Build history of the part. All positions in model axes, mm. A direction names the side the tool comes from. Give positions to 0.01 mm unless a question says otherwise; leave off trailing zeros. Order: outer loops, then holes, each group sorted by start corner. A loop starts at its lowest first (then second) coordinate and runs counter-clockwise, first axis right, second up. Notation, with made-up numbers: (24, 81.5) - (65, 81.5) arc R24 cw to (65, 119.5) - close; hole circle Ø4 at (79, 44.25). An arc over 180 degrees is marked (long way). Use a Markdown table: item, result. Add a question column.
(1) Slice it at A-A (y = 0). Write the cut outline in (x, z).
(2) Slice it at C-C (z = -12). Write the cut outline in (x, y), then the cut area to 3 significant figures.
(3) Wall check: line 1 (Y direction, x = 0, z = -9.5); line 2 (Z direction, x = -30.5, y = -13); line 3 (Y direction, x = 5.5, z = -12.25). Give the ranges that are in metal, low to high.
(4) Which spindle directions (+Z, -Z, +X, -X, +Y, -Y) get a long thin tool onto all of the face, cutting with end or side? Do faces 5 (the face through (-14, -28, -18.5)), 6 (the face through (22.41, 17.47, 1.93)). Say none if no direction does.
(5) Mould opens along X. For faces 1 (the face through (-25.39, -25.52, -16.04)), 2 (the face through (36, 0, -16)), 3 (the face through (-4.81, 21.15, 5.5)), 4 (the face through (-23.866, -16.582, 1.873)) say: +X half, -X half, draft (parallel to the pull), parting line (faces both ways), or undercut.
(6) Flat gauge pins, fed straight in: pin 1 (4 mm diameter, centred on x = -33.26, y = -13.78, fed in from +Z); pin 2 (1.8 mm diameter, centred on x = -13.78, y = 33.26, fed in from +Z); pin 3 (4 mm diameter, centred on y = 16, z = -1.5, fed in from -X); pin 4 (8 mm diameter, centred on y = -17, z = 2.5, fed in from +X). Where does each tip first touch, or does it go through?
from build123d import *

# Parameters (mm, degrees)
SKETCH_2_R                = 32.5
SKETCH_2_R_2              = 1.5
SKETCH_2_R_3              = 21
EXTRUDE_1_DEPTH           = 5.5
SKETCH_3_R                = 32.5
SKETCH_3_R_2              = 30.5
EXTRUDE_2_DEPTH           = 18.5
SKETCH_4_R                = 1.5
SKETCH_4_R_2              = 30.5
EXTRUDE_3_DEPTH           = 5.5
CHAMFER_1_SIZE            = 1
CHAMFER_3_SIZE            = 0.5
HOLE_WIZARD_0_D           = 3.2
HOLE_WIZARD_0_DEPTH       = 8.1
HOLE_WIZARD_0_CSINK_D     = 6.6
HOLE_WIZARD_0_CSINK_ANGLE = 90
HOLE_WIZARD_0_TIP         = 0.96137699
HOLE_WIZARD_1_D           = 3.2
HOLE_WIZARD_1_DEPTH       = 8.1
HOLE_WIZARD_1_CSINK_D     = 6.6
HOLE_WIZARD_1_CSINK_ANGLE = 90
HOLE_WIZARD_1_TIP         = 0.96137699


with BuildPart() as part:
    # 草图2 → 凸台-拉伸1 (new body)
    with BuildSketch(Plane.XY):
        Circle(SKETCH_2_R)
        with Locations((-15.969331282, -22.388176755)):
            Circle(SKETCH_2_R_2, mode=Mode.SUBTRACT)
        with Locations((-22.388176755, -15.969331282)):
            Circle(SKETCH_2_R_2, mode=Mode.SUBTRACT)
        with Locations((-22.388176755, 15.969331282)):
            Circle(SKETCH_2_R_2, mode=Mode.SUBTRACT)
        with Locations((-15.969331282, 22.388176755)):
            Circle(SKETCH_2_R_2, mode=Mode.SUBTRACT)
        with Locations((15.969331282, 22.388176755)):
            Circle(SKETCH_2_R_2, mode=Mode.SUBTRACT)
        with Locations((22.388176755, 15.969331282)):
            Circle(SKETCH_2_R_2, mode=Mode.SUBTRACT)
        with Locations((22.388176755, -15.969331282)):
            Circle(SKETCH_2_R_2, mode=Mode.SUBTRACT)
        with Locations((15.969331282, -22.388176755)):
            Circle(SKETCH_2_R_2, mode=Mode.SUBTRACT)
        Circle(SKETCH_2_R_3, mode=Mode.SUBTRACT)
    extrude(amount=EXTRUDE_1_DEPTH)

    # 草图3 → 凸台-拉伸2 (add)
    with BuildSketch(Plane(origin=(0, 0, 0), x_dir=(-1, 0, 0), z_dir=(0, 0, -1))):
        Circle(SKETCH_3_R)
        Circle(SKETCH_3_R_2, mode=Mode.SUBTRACT)
    extrude(amount=EXTRUDE_2_DEPTH)

    # 草图4 → 凸台-拉伸3 (add)
    with BuildSketch(Plane(origin=(0, 0, -18.5), x_dir=(-1, 0, 0), z_dir=(0, 0, -1))):
        with BuildLine():
            ThreePointArc((-10.328522738, 36.591619506), (-15.498679334, 37.417120933), (-18.570814392, 33.177550434))
            ThreePointArc((-18.570814392, 33.177550434), (-19.210808968, 31.084296828), (-20.683639012, 29.465014462))
            ThreePointArc((-20.683639012, 29.465014462), (-25.455844342, 25.455843903), (-29.465014819, 20.683638503))
            ThreePointArc((-29.465014819, 20.683638503), (-31.084297159, 19.210808432), (-33.177550755, 18.570813819))
            ThreePointArc((-33.177550755, 18.570813819), (-37.4171212, 15.498678688), (-36.591619684, 10.328522106))
            ThreePointArc((-36.591619684, 10.328522106), (-35.564010369, 8.395823782), (-35.460452938, 6.209370129))
            ThreePointArc((-35.460452938, 6.209370129), (-36, -3.11e-07), (-35.460452831, -6.209370741))
            ThreePointArc((-35.460452831, -6.209370741), (-35.564010224, -8.395824396), (-36.591619506, -10.328522738))
            ThreePointArc((-36.591619506, -10.328522738), (-37.417120933, -15.498679334), (-33.177550434, -18.570814392))
            ThreePointArc((-33.177550434, -18.570814392), (-31.084296828, -19.210808968), (-29.465014462, -20.683639012))
            ThreePointArc((-29.465014462, -20.683639012), (-25.455843903, -25.455844342), (-20.683638503, -29.465014819))
            ThreePointArc((-20.683638503, -29.465014819), (-19.210808432, -31.084297159), (-18.57081382, -33.177550755))
            ThreePointArc((-18.57081382, -33.177550755), (-15.498678688, -37.4171212), (-10.328522106, -36.591619684))
            ThreePointArc((-10.328522106, -36.591619684), (-8.395823782, -35.564010369), (-6.209370129, -35.460452938))
            ThreePointArc((-6.209370129, -35.460452938), (3.11e-07, -36), (6.209370741, -35.460452831))
            ThreePointArc((6.209370741, -35.460452831), (8.395824396, -35.564010224), (10.328522738, -36.591619506))
            ThreePointArc((10.328522738, -36.591619506), (15.498679334, -37.417120933), (18.570814392, -33.177550434))
            ThreePointArc((18.570814392, -33.177550434), (19.210808968, -31.084296828), (20.683639012, -29.465014462))
            ThreePointArc((20.683639012, -29.465014462), (25.455844342, -25.455843903), (29.465014819, -20.683638503))
            ThreePointArc((29.465014819, -20.683638503), (31.084297159, -19.210808432), (33.177550755, -18.57081382))
            ThreePointArc((33.177550755, -18.57081382), (37.4171212, -15.498678688), (36.591619684, -10.328522106))
            ThreePointArc((36.591619684, -10.328522106), (35.564010369, -8.395823782), (35.460452938, -6.209370129))
            ThreePointArc((35.460452938, -6.209370129), (36, 3.11e-07), (35.460452831, 6.209370741))
            ThreePointArc((35.460452831, 6.209370741), (35.564010224, 8.395824396), (36.591619506, 10.328522738))
            ThreePointArc((36.591619506, 10.328522738), (37.417120933, 15.498679334), (33.177550434, 18.570814392))
            ThreePointArc((33.177550434, 18.570814392), (31.084296828, 19.210808968), (29.465014462, 20.683639012))
            ThreePointArc((29.465014462, 20.683639012), (25.455843903, 25.455844342), (20.683638503, 29.465014819))
            ThreePointArc((20.683638503, 29.465014819), (19.210808432, 31.084297159), (18.57081382, 33.177550755))
            ThreePointArc((18.57081382, 33.177550755), (15.498678688, 37.4171212), (10.328522106, 36.591619684))
            ThreePointArc((10.328522106, 36.591619684), (8.395823782, 35.564010369), (6.209370129, 35.460452938))
            ThreePointArc((6.209370129, 35.460452938), (-3.11e-07, 36), (-6.209370741, 35.460452831))
            ThreePointArc((-6.209370741, 35.460452831), (-8.395824396, 35.564010224), (-10.328522738, 36.591619506))
        make_face()
        with Locations((-13.776603852, 33.259663052)):
            Circle(SKETCH_4_R, mode=Mode.SUBTRACT)
        with Locations((13.776603278, 33.259663289)):
            Circle(SKETCH_4_R, mode=Mode.SUBTRACT)
        with Locations((33.259663052, 13.776603852)):
            Circle(SKETCH_4_R, mode=Mode.SUBTRACT)
        with Locations((33.259663289, -13.776603278)):
            Circle(SKETCH_4_R, mode=Mode.SUBTRACT)
        with Locations((13.776603852, -33.259663052)):
            Circle(SKETCH_4_R, mode=Mode.SUBTRACT)
        with Locations((-13.776603278, -33.259663289)):
            Circle(SKETCH_4_R, mode=Mode.SUBTRACT)
        with Locations((-33.259663052, -13.776603852)):
            Circle(SKETCH_4_R, mode=Mode.SUBTRACT)
        with Locations((-33.259663289, 13.776603278)):
            Circle(SKETCH_4_R, mode=Mode.SUBTRACT)
        Circle(SKETCH_4_R_2, mode=Mode.SUBTRACT)
    extrude(amount=-EXTRUDE_3_DEPTH)

    # 倒角1
    chamfer_1_edges = [part.edges().sort_by_distance(p)[0] for p in [
        (-32.5, 0, 5.5),
    ]]
    chamfer(chamfer_1_edges, length=CHAMFER_1_SIZE)

    # 倒角3
    chamfer_3_edges = [part.edges().sort_by_distance(p)[0] for p in [
        (-21, 0, 5.5),
        (30.5, 0, -18.5),
        (8.395824396, 35.564010224, -13),
        (3.11e-07, 36, -13),
        (-8.395823782, 35.564010369, -13),
        (-15.498678688, 37.4171212, -13),
        (-19.210808432, 31.084297159, -13),
        (-25.455843903, 25.455844342, -13),
        (-31.084296828, 19.210808968, -13),
        (-37.417120933, 15.498679334, -13),
        (-35.564010224, 8.395824396, -13),
        (-36, 3.11e-07, -13),
        (-35.564010369, -8.395823782, -13),
        (-37.4171212, -15.498678688, -13),
        (-31.084297159, -19.210808432, -13),
        (-25.455844342, -25.455843903, -13),
        (-19.210808968, -31.084296828, -13),
        (-15.498679334, -37.417120933, -13),
        (-8.395824396, -35.564010224, -13),
        (-3.11e-07, -36, -13),
        (8.395823782, -35.564010369, -13),
        (15.498678688, -37.4171212, -13),
        (19.210808432, -31.084297159, -13),
        (25.455843903, -25.455844342, -13),
        (31.084296828, -19.210808968, -13),
        (37.417120933, -15.498679334, -13),
        (35.564010224, -8.395824396, -13),
        (36, -3.11e-07, -13),
        (35.564010369, 8.395823782, -13),
        (37.4171212, 15.498678688, -13),
        (31.084297159, 19.210808432, -13),
        (25.455844342, 25.455843903, -13),
        (19.210808968, 31.084296828, -13),
        (15.498679334, 37.417120933, -13),
    ]]
    chamfer(chamfer_3_edges, length=CHAMFER_3_SIZE)

    # 打孔尺寸(%根据十字)槽沉头木螺钉的类型0
    with Locations(Plane.XY.offset(-13)):
        with Locations((13.776603852, 33.259663052), (33.259663052, -13.776603852), (-13.776603852, -33.259663052), (-33.259663052, 13.776603852)):
            CounterSinkHole(HOLE_WIZARD_0_D / 2, HOLE_WIZARD_0_CSINK_D / 2, depth=HOLE_WIZARD_0_DEPTH, counter_sink_angle=HOLE_WIZARD_0_CSINK_ANGLE)
            with Locations((0, 0, -(HOLE_WIZARD_0_DEPTH + HOLE_WIZARD_0_TIP / 2))):  # 118° drill point
                Cone(0, HOLE_WIZARD_0_D / 2, HOLE_WIZARD_0_TIP, mode=Mode.SUBTRACT)

    # 打孔尺寸(%根据十字)槽沉头木螺钉的类型1
    with Locations(Plane.XY.offset(5.5)):
        with Locations((-15.969331282, 22.388176755), (-22.388176755, 15.969331282), (-22.388176755, -15.969331282), (-15.969331282, -22.388176755), (15.969331282, -22.388176755), (22.388176755, -15.969331282), (22.388176755, 15.746279838), (15.969331282, 22.388176755)):
            CounterSinkHole(HOLE_WIZARD_1_D / 2, HOLE_WIZARD_1_CSINK_D / 2, depth=HOLE_WIZARD_1_DEPTH, counter_sink_angle=HOLE_WIZARD_1_CSINK_ANGLE)
            with Locations((0, 0, -(HOLE_WIZARD_1_DEPTH + HOLE_WIZARD_1_TIP / 2))):  # 118° drill point
                Cone(0, HOLE_WIZARD_1_D / 2, HOLE_WIZARD_1_TIP, mode=Mode.SUBTRACT)


solid = part.part
Solution:
| question | item | result |
|---|---|---|
| 1 | outline | (-36, -18.5) - (-31, -18.5) - (-30.5, -18) - (-30.5, 0) - (-21, 0) - (-21, 5) - (-21.5, 5.5) - (-31.5, 5.5) - (-32.5, 4.5) - (-32.5, -13) - (-35.5, -13) - (-36, -13.5) - close; (21, 0) - (30.5, 0) - (30.5, -18) - (31, -18.5) - (36, -18.5) - (36, -13.5) - (35.5, -13) - (32.5, -13) - (32.5, 4.5) - (31.5, 5.5) - (21.5, 5.5) - (21, 5) - close |
| 2 | outline | circle Ø65 at (0, 0); hole circle Ø61 at (0, 0) |
| 2 | area | 396 mm2 |
| 3 | line 1 | -32.5 to -30.5, 30.5 to 32.5 |
| 3 | line 2 | -18.5 to -13 |
| 3 | line 3 | -32.03 to -30, 30 to 32.03 |
| 4 | face 5 | -Z, +X, -X, +Y, -Y |
| 4 | face 6 | +Z, -Z |
| 5 | face 1 | -X half |
| 5 | face 2 | +X half |
| 5 | face 3 | draft |
| 5 | face 4 | undercut |
| 6 | pin 1 | z = -13 |
| 6 | pin 2 | through |
| 6 | pin 3 | x = -29.33 |
| 6 | pin 4 | x = 29.79 |
